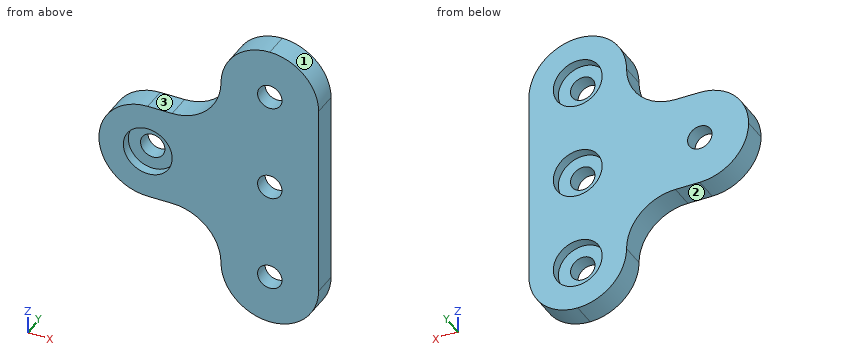
```python
from build123d import *

# Parameters (mm, degrees)
F1_DEPTH       = 5
F2_D           = 5
F2_CBORE_D     = 10
F2_CBORE_DEPTH = 2
F3_R           = 9.99999
F5_D           = 5
F5_CBORE_D     = 10
F5_CBORE_DEPTH = 2


# Not quite as in the source:
# - a fillet or chamfer is up to 0.001 mm smaller than in the source, because OpenCascade refuses the exact size


with BuildPart() as f1:
    # F0 (on Front) → F1 (new body)
    with BuildSketch(Plane.XZ):
        Polygon((15, 10), (-10, 10), (-10, -10), (15, -10), (15, -30), (35, -30), (35, -10), (35, 10), (35, 30), (15, 30), align=None)
    extrude(amount=F1_DEPTH)

    # F2 (through all)
    with Locations(Plane(origin=(0, 0, 0), x_dir=(1, 0, 0), z_dir=(0, 1, 0))):
        with Locations((25, -20), (25, 20), (25, 0)):
            CounterBoreHole(F2_D / 2, F2_CBORE_D / 2, F2_CBORE_DEPTH)

    # F3 (radius 10 in the source; OpenCascade refuses exactly that, so slightly less here)
    f3_edges = [f1.edges().sort_by_distance(p)[0] for p in [
        (35, -2.5, 30),
        (35, -2.5, -30),
        (15, -2.5, -30),
        (15, -2.5, 30),
        (-10, -2.5, 10),
        (-10, -2.5, -10),
        (15, -2.5, 10),
        (15, -2.5, -10),
    ]]
    fillet(f3_edges, radius=F3_R)

    # F5 (through all)
    with Locations(Plane.XZ.offset(5)):
        with Locations((0, 0)):
            CounterBoreHole(F5_D / 2, F5_CBORE_D / 2, F5_CBORE_DEPTH)


solid = f1.part
```
Read the model definition and answer for the solid it produces. Units are mm, in the model's axes. Face numbers are marked on the shaded views. A direction names the side the tool comes from. Give positions to 0.01 mm unless a question says otherwise; leave off trailing zeros. Loops run counter-clockwise (first coordinate to the right, second up) from the corner with the lowest first, then second, coordinate; pieces in that order, holes last.
Item 1: The part is cut by section C-C (z = 16). Write down the section's boundary in (x, y), and give its area (3 significant figures).
Item 2: The part is cut by section A-A (y = -4.1). Give the number of separate pieces and of enclosed holes in the cut face, and give its area (3 significant figures).
Item 3: Each of these flat-tipped pins is pushed along its axis until it touches: pin 1 Ø5 at (x, z) = (24, -2) entering from +Y; pin 2 Ø4.5 at (x, z) = (25, -20) entering from -Y; pin 3 Ø1.5 at (x, y) = (3, -3) entering from -Z; pin 4 Ø3 at (x, y) = (-4, -3) entering from +Z. Where does it stop, or does it pass through?
Item 4: Find the intervals of material crossed by line 1 along Z through (x, y) = (25, -1.1); line 2 along X through (y, z) = (-3.15, -20); line 3 along Z through (x, y) = (26, -1.75), in increasing order.
Item 5: The part is cut by section B-B (x = -1.5). Write down the section's boundary in (y, z).
Item 6: For the marked faces 1, 2 and 3, determine the directions among +Z, -Z, +X, -X, +Y, -Y from which every point of the face is accessible in a straight line to the end or side of a thin tool.
Taken from the geometry:
1. outline: (14.17, -5) - (35, -5) - (35, 0) - (28, 0) - (28, -2) - (22, -2) - (22, 0) - (14.17, 0) - close
1. area: 92.2 mm2
2. separate pieces: 1
2. enclosed holes: 4
2. area: 1,480 mm2
3. pin 1: stops at y = -2
3. pin 2: passes through
3. pin 3: stops at z = -10
3. pin 4: stops at z = 9.68
4. line 1: z = -30 to -25, -15 to -5, 5 to 15, 25 to 30
4. line 2: x = 15 to 22.5, 27.5 to 35
4. line 3: z = -29.95 to -24.9, -15.1 to -4.9, 4.9 to 15.1, 24.9 to 29.95
5. outline: (-5, -9.89) - (0, -9.89) - (0, -2) - (-3, -2) - (-3, -4.77) - (-5, -4.77) - close; (-5, 4.77) - (-3, 4.77) - (-3, 2) - (0, 2) - (0, 9.89) - (-5, 9.89) - close
6. face 1: +Z, +X, +Y, -Y
6. face 2: -Z, -X, +Y, -Y
6. face 3: +Z, -X, +Y, -Y
